Work out the finished part from the listing and answer in its coordinate system (mm). A direction names the side the tool comes from. Round coordinates to 2 decimals unless told otherwise and drop trailing zeros. Order: outer loops, then holes, each group sorted by start corner. A loop starts at its lowest first (then second) coordinate and runs counter-clockwise, first axis right, second up. Notation, with made-up numbers: (68, -12) - (87, -12) arc R28 cw to (87, 12) - close; hole circle Ø3 at (-9.75, 28). An arc over 180 degrees is marked (long way). Answer in a Markdown table with one row per item.
from build123d import *

# Parameters (mm, degrees)
SKETCH1_R           = 9.667215137
BOSS_EXTRUDE1_DEPTH = 50.8
SKETCH2_W           = 19.334430274
SKETCH2_H           = 12.7
BOSS_EXTRUDE2_DEPTH = 8.89
BOSS_EXTRUDE3_DEPTH = 25.4
SKETCH5_W           = 0.549916313
SKETCH5_H           = 38.1
BOSS_EXTRUDE4_DEPTH = 25.4
SKETCH6_W           = 25.4
SKETCH6_H           = 6.473300788
BOSS_EXTRUDE5_DEPTH = 25.4
BOSS_EXTRUDE6_DEPTH = 8.89
BOSS_EXTRUDE7_START = 5.08
BOSS_EXTRUDE7_DEPTH = 5.08


with BuildPart() as part:
    # Sketch1 → Boss-Extrude1 (new body)
    with BuildSketch(Plane.XY):
        Circle(SKETCH1_R)
    extrude(amount=BOSS_EXTRUDE1_DEPTH)

    # Sketch2 → Boss-Extrude2 (add)
    with BuildSketch(Plane(origin=(0, 0, 0), x_dir=(-1, 0, 0), z_dir=(0, 0, -1))):
        with Locations((0, 6.35)):
            Rectangle(SKETCH2_W, SKETCH2_H)
    extrude(amount=-BOSS_EXTRUDE2_DEPTH)

    # Sketch4 → Boss-Extrude3 (add)
    with BuildSketch(Plane(origin=(0, 0, 0), x_dir=(-1, 0, 0), z_dir=(0, 0, -1))):
        Polygon((-31.75, 12.7), (-31.75, 22.935187234), (31.75, 22.935187234), (31.75, 12.7), (9.667215137, 12.7), (-9.667215137, 12.7), align=None)
    extrude(amount=-BOSS_EXTRUDE3_DEPTH)

    # Sketch5 → Boss-Extrude4 (add)
    with BuildSketch(Plane(origin=(0, 0, 0), x_dir=(-1, 0, 0), z_dir=(0, 0, -1))):
        with Locations((31.475041844, 41.985187234)):
            Rectangle(SKETCH5_W, SKETCH5_H)
        with Locations((-31.475041844, 41.985187234)):
            Rectangle(SKETCH5_W, SKETCH5_H)
    extrude(amount=-BOSS_EXTRUDE4_DEPTH)

    # Sketch6 → Boss-Extrude5 (add)
    with BuildSketch(Plane(origin=(0, 0, 0), x_dir=(-1, 0, 0), z_dir=(0, 0, -1))):
        with Locations((19.05, 64.271837628)):
            Rectangle(SKETCH6_W, SKETCH6_H)
        with Locations((-19.05, 64.271837628)):
            Rectangle(SKETCH6_W, SKETCH6_H)
    extrude(amount=-BOSS_EXTRUDE5_DEPTH)

    # Sketch7 → Boss-Extrude6 (add)
    with BuildSketch(Plane(origin=(0, 0, 0), x_dir=(-1, 0, 0), z_dir=(0, 0, -1))):
        Polygon((-31.75, 12.7), (-9.667215137, 0), (-9.667215137, 2.54), (-29.21, 12.7), align=None)
        Polygon((9.667215137, 0), (31.75, 12.7), (29.21, 12.7), (9.667215137, 2.54), align=None)
    extrude(amount=-BOSS_EXTRUDE6_DEPTH)

    # Sketch14 → Boss-Extrude7 (add)
    with BuildSketch(Plane(origin=(0, 0, 0), x_dir=(-1, 0, 0), z_dir=(0, 0, -1)).offset(BOSS_EXTRUDE7_START)):
        with BuildLine():
            Line((9.667215137, 22.935187234), (-9.667215137, 22.935187234))
            Line((-9.667215137, 22.935187234), (-9.667215137, 0))
            ThreePointArc((-9.667215137, 0), (0, -9.667215137), (9.667215137, 0))
            Line((9.667215137, 0), (9.667215137, 22.935187234))
        make_face()
    extrude(amount=-BOSS_EXTRUDE7_DEPTH)


solid = part.part
1) Find section C-C, the plane y = 29. Give the vertices of the cut face in (x, z), then the cut area to 3 significant figures.
Filled in:
| item | result |
|---|---|
| outline | (-31.75, 0) - (-31.2, 0) - (-31.2, 25.4) - (-31.75, 25.4) - close; (31.2, 0) - (31.75, 0) - (31.75, 25.4) - (31.2, 25.4) - close |
| area | 27.9 mm^2 |
2) Which of the six approach directions +Z, -Z, +X, -X, +Y, -Y give full straight-line access (tool end or side, diameter ignored) to faces 1 (the face through (19.3, 7.55, 4.38)), 2 (the face through (-2, 22, 25.4)), 3 (the face through (6.35, 64, 13))?
Filled in:
| item | result |
|---|---|
| face 1 | +Z, -Z |
| face 2 | +Z, +X, -X, +Y |
| face 3 | +Z, -Z, +Y |
3) Find section A-A, the plane z = 18.5. Give the vertices of the cut face in (x, y).
Filled in:
| item | result |
|---|---|
| outline | (-31.75, 12.7) - (31.75, 12.7) - (31.75, 67.51) - (6.35, 67.51) - (6.35, 61.04) - (31.2, 61.04) - (31.2, 22.94) - (-31.2, 22.94) - (-31.2, 61.04) - (-6.35, 61.04) - (-6.35, 67.51) - (-31.75, 67.51) - close; circle Ø19.33 at (0, 0) |
4) Find section D-D, the plane x = -16.5. Give the vertices of the cut face in (y, z), then the cut area to 3 significant figures.
Filled in:
| item | result |
|---|---|
| outline | (3.93, 0) - (6.09, 0) - (6.09, 8.89) - (3.93, 8.89) - close; (12.7, 0) - (22.94, 0) - (22.94, 25.4) - (12.7, 25.4) - close; (61.04, 0) - (67.51, 0) - (67.51, 25.4) - (61.04, 25.4) - close |
| area | 444 mm^2 |
5) Each of these flat-tipped pins is pushed along its axis until it touches: pin 1 (20.5 mm diameter, centred on x = -22.5, y = 49.5, fed in from -Z); pin 2 (12 mm diameter, centred on x = 24, y = 26.5, fed in from +Z); pin 3 (10 mm diameter, centred on x = 1, z = 17, fed in from -Y); pin 4 (7.5 mm diameter, centred on x = -18, z = 18.5, fed in from -Y). Where does it stop, or does it pass through?
Filled in:
| item | result |
|---|---|
| pin 1 | stops at z = 0 |
| pin 2 | stops at z = 25.4 |
| pin 3 | stops at y = -9.67 |
| pin 4 | stops at y = 12.7 |
6) Find the intervals of material crossed by probe 1 along X at (y, z) = (32, 23.5); probe 2 along Y at (x, z) = (-7, 11); probe 3 along X at (y, z) = (63, 16), in increasing order. Write a range as from..to.
Filled in:
| item | result |
|---|---|
| probe 1 | x = -31.75..-31.2, 31.2..31.75 |
| probe 2 | y = -6.67..6.67, 12.7..22.94, 61.04..67.51 |
| probe 3 | x = -31.75..-6.35, 6.35..31.75 |
7) Find section B-B, the plane z = 3. Give the vertices of the cut face in (x, y), then the cut area to 3 significant figures.
Filled in:
| item | result |
|---|---|
| outline | (-31.75, 12.7) - (-9.67, 0) arc R9.67 ccw to (9.67, 0) - (31.75, 12.7) - (31.75, 67.51) - (6.35, 67.51) - (6.35, 61.04) - (31.2, 61.04) - (31.2, 22.94) - (-31.2, 22.94) - (-31.2, 61.04) - (-6.35, 61.04) - (-6.35, 67.51) - (-31.75, 67.51) - close; hole (-29.21, 12.7) - (-9.67, 2.54) - (-9.67, 12.7) - close; hole (9.67, 2.54) - (29.21, 12.7) - (9.67, 12.7) - close |
| area | 1,490 mm^2 |
8) The mould has two halves that part along Y. Classify faces 4 (the face through (19, 67.508, 13)), 5 (the face through (-6.35, 64, 13)), 6 (the face through (31.2, 42, 13)), 7 (the face through (-9.667, 9, 0)): released by +Y, released by -Y, zero draft, split by the parting line, or undercut.
Filled in:
| item | result |
|---|---|
| face 4 | released by +Y |
| face 5 | zero draft |
| face 6 | undercut |
| face 7 | undercut |
